Geometry check sheet. Reference: the model listing, model coordinates, mm. A direction names the side the tool comes from. Coordinates: 2 decimals unless noted, no trailing zeros. Write each loop counter-clockwise with the first axis right and the second up, starting at its lowest first coordinate (ties: lowest second). Pieces come first, ordered by that corner, then holes. Notation, with made-up numbers: (76.5, 26) -> (98.5, 26) arc R21 cw to (98.5, 46) -> close; hole circle Ø6 at (79, 67.5). An arc over 180 degrees is marked (long way). Answer in a Markdown table with one row per item. Add a question column.
1. Cross-section at A-A on z = -8.5. Record the cut outline in (x, y).
2. Set-up check for faces 4 (the flat face through (-24.344, 1.479, -19.229)), 5 (the flat face through (-14, 3, -23)): record each of +Z, -Z, +X, -X, +Y, -Y from which the full face is reachable in a straight line by a thin tool's end or side.
3. Depth check by flat-ended pin: P1, Ø5, axis at x = -25, z = -9.5, coming from the +Y side. Enter the tip coordinate at first touch or a pass-through.
4. Cross-section at C-C on y = 1.1. Record the cut outline in (x, z), and give its area (3 significant figures).
5. Cross-section at B-B on x = -26. Record the cut outline in (y, z), and give its area (3 significant figures).
6. Scan lines: L1, parallel to X at y = 2.8, z = -12; L2, parallel to X at y = 2.8, z = -23.5; L3, parallel to Z at x = -1, y = 1.6. Record each from-to range of solid material in increasing order. Write a range as from..to.
7. Mould release check, pull along X, two halves, no side actions. Record for faces 1 (the flat face through (-15, 1, -29.8)), 2 (the flat face through (3, 1, -12)), 3 (the flat face through (-22, 1, -27.15)): pulls with the +X half, pulls with the -X half, needs draft (parallel to the pull), parting line crosses it, or undercut.
Autodesk Inventor part; units mm, degrees
ref_plane "YZ Plane" through (0, 0, 0) normal (1, 0, 0) x (0, 1, 0)
ref_plane "XZ Plane" through (0, 0, 0) normal (0, 1, 0) x (-1, 0, 0)
ref_plane "XY Plane" through (0, 0, 0) normal (0, 0, 1) x (1, 0, 0)
sketch "Sketch1" plane through (0, 0, 0) normal (0, 1, 0) x (-1, 0, 0)
  line L0 (0, 0) -> (20.8, 0)
  line L1 (20.8, 0) -> (20.8, -22.6) construction
  line L2 (20.8, -22.6) -> (0, -22.6)
  line L3 (0, -22.6) -> (0, 0)
  line L4 (22.8, 4.35) -> (20.8, 4.35)
  line L5 (20.8, -26.95) -> (22.8, -26.95)
  line L6 (24.6, 0.15) -> (24.6, -22.45) construction
  line L7 (29.6, -14.7432) -> (24.6, -14.7432)
  line L8 (24.6, -14.7432) -> (24.6, 0.15) construction
  line L9 (24.6, -14.7432) -> (22.8, -14.7432) construction
  line L10 (24.6, -15.7432) -> (22.8, -15.7432) construction
  line L11 (24.6, -15.7432) -> (23.7, -22.6)
  line L12 (0, 0) -> (0, 7.2) construction
  line L13 (0, 7.2) -> (-3, 7.2) construction
  line L14 (-3, 7.2) -> (32, 7.2)
  line L15 (32, 7.2) -> (32, -29.8)
  line L16 (32, -29.8) -> (-3, -29.8)
  line L17 (-3, -29.8) -> (-3, 7.2)
  line L18 (24.6, 0.15) -> (24.6, -15.7432) construction
  line L19 (22.8, -22.6) -> (23.7, -22.6)
  line L20 (22.8, 0.1568) -> (22.8, 4.35)
  line L21 (22.8, -26.95) -> (22.8, -22.6)
  line L22 (24.6, -14.7432) -> (24.6, -15.7432)
  line L23 (20.8, 4.35) -> (20.8, 0)
  line L24 (20.8, -22.6) -> (20.8, -26.95)
  line L25 (29.6, 0.1568) -> (29.6, -14.7432)
  line L26 (22.8, 0.1568) -> (29.6, 0.1568)
  line L27 (29.8, 0.3568) -> (29.8, -14.9432)
  line L28 (29.8, -14.9432) -> (24.8, -14.9432)
  line L29 (24.8, -14.9432) -> (24.8, -15.7563)
  line L30 (24.8, -15.7563) -> (23.8755, -22.8)
  line L31 (23.8755, -22.8) -> (23, -22.8)
  line L32 (23, -22.8) -> (23, -27.15)
  line L33 (23, -27.15) -> (20.6, -27.15)
  line L34 (20.6, -27.15) -> (20.6, -22.8)
  line L35 (20.6, -22.8) -> (-0.2, -22.8)
  line L36 (-0.2, -22.8) -> (-0.2, 0.2)
  line L37 (-0.2, 0.2) -> (20.6, 0.2)
  line L38 (20.6, 0.2) -> (20.6, 4.55)
  line L39 (20.6, 4.55) -> (23, 4.55)
  line L40 (23, 4.55) -> (23, 0.3568)
  line L41 (23, 0.3568) -> (29.8, 0.3568)
  point P0 (20.8, -11.3)
  dimension "d0" = 20.8
  dimension "d1" = 22.6
  dimension "d2" = 2
  dimension "d5" = 22.6
  dimension "d8" = 1
  dimension "d9" = 7.2
  dimension "d10" = 3
  dimension "d11" = 35
  dimension "d12" = 37
  dimension "d16" = 2
  dimension "d19" = 4.35
  dimension "d26" = 6.8
  dimension "d27" = 0.9
  dimension "d28" = 14.9
  dimension "d29" = 5
  dimension "d32" = 0.2
  dimension "d35" = 4.35
extrude "Extrusion5" add sketch "Sketch1" along normal blind 3 contours L14 L15 L16 L17
properties part number "flipper_robot_v2_servo_side_profile"
Results found:
| question | item | result |
|---|---|---|
| 1 | outline | (-32, 0) -> (-29.8, 0) -> (-29.8, 3) -> (-32, 3) -> close; (0.2, 0) -> (3, 0) -> (3, 3) -> (0.2, 3) -> close |
| 2 | face 4 | +Y, -Y |
| 2 | face 5 | +Z, -Z, +X, -X, +Y |
| 3 | P1 | passes through |
| 4 | outline | (-32, -29.8) -> (3, -29.8) -> (3, 7.2) -> (-32, 7.2) -> close; hole (-29.8, -14.94) -> (-24.8, -14.94) -> (-24.8, -15.76) -> (-23.88, -22.8) -> (-23, -22.8) -> (-23, -27.15) -> (-20.6, -27.15) -> (-20.6, -22.8) -> (0.2, -22.8) -> (0.2, 0.2) -> (-20.6, 0.2) -> (-20.6, 4.55) -> (-23, 4.55) -> (-23, 0.36) -> (-29.8, 0.36) -> close |
| 4 | area | 626 mm^2 |
| 5 | outline | (0, -29.8) -> (3, -29.8) -> (3, -14.94) -> (0, -14.94) -> close; (0, 0.36) -> (3, 0.36) -> (3, 7.2) -> (0, 7.2) -> close |
| 5 | area | 65.1 mm^2 |
| 6 | L1 | x = -32..-29.8, 0.2..3 |
| 6 | L2 | x = -32..-23, -20.6..3 |
| 6 | L3 | z = -29.8..-22.8, 0.2..7.2 |
| 7 | face 1 | needs draft |
| 7 | face 2 | pulls with the +X half |
| 7 | face 3 | undercut |
